Can you work these out from the model? Positions are in its coordinate system, mm. Round coordinates to 2 decimals unless told otherwise and drop trailing zeros. Write each loop counter-clockwise with the first axis right and the second up, starting at its lowest first coordinate (ties: lowest second). Pieces come first, ordered by that corner, then holes. Notation, with made-up numbers: (-23.5, -39.5) -> (4.5, -39.5) arc R22 ccw to (4.5, -31.5) -> close; hole circle Ø7 at (2, 13). An arc over 180 degrees is marked (long way). Write item = value, one per line. Start each with the question number.
1) Imagine slicing it at A-A, the plane y = -115.57. Please give me the cut outline in (x, z) (3 decimals).
2) Imagine slicing it at C-C, the plane z = 0.25. State how many separate pieces and enclosed holes the cut face has, then the cut area to 3 significant figures.
3) Thinking about a two-plate mould opening in X: for faces 1 (the face through (109.159, -124.952, 0.789)), 2 (the face through (125, -113, 0)), 3 (the face through (141.82, -104.477, 0.789)), which applies, +X half, -X half, draft (parallel to the pull), parting line (faces both ways), or undercut?
4) Imagine slicing it at B-B, the plane x = 111.76. Please give me the cut outline in (y, z).
5) If I drill on line 1 (X direction, y = -115.57, z = 1.35) (3 decimals); line 2 (X direction, y = -121.5, z = 0.6); line 3 (Y direction, x = 131, z = 0.4), over which ranges is the centre line in solid material (lowest first)?
Autodesk Inventor part; units mm, degrees
ref_plane "Plan YZ" through (0, 0, 0) normal (1, 0, 0) x (0, 1, 0)
ref_plane "Plan XZ" through (0, 0, 0) normal (0, 1, 0) x (-1, 0, 0)
ref_plane "Plan XY" through (0, 0, 0) normal (0, 0, 1) x (1, 0, 0)
sketch "Esquisse1" plane through (0, 0, 0) normal (0, 0, 1) x (1, 0, 0)
  point P0 (0, 0)
sketch "Esquisse6" plane through (0, 0, 0) normal (0, 0, 1) x (1, 0, 0)
  arc A0 (111.379, -99.822) -> (108.204, -102.997) centre (111.379, -102.997) ccw
  line L0 (108.204, -102.997) -> (108.204, -122.682)
  arc A1 (108.204, -122.682) -> (111.379, -125.857) centre (111.379, -122.682) ccw
  line L1 (111.379, -125.857) -> (139.954, -125.857)
  arc A2 (139.954, -125.857) -> (143.129, -122.682) centre (139.954, -122.682) ccw
  line L2 (143.129, -122.682) -> (143.129, -102.997)
  arc A3 (143.129, -102.997) -> (139.954, -99.822) centre (139.954, -102.997) ccw
  line L3 (139.954, -99.822) -> (111.379, -99.822)
  circle A4 centre (120.269, -122.428) radius 0.4
  circle A5 centre (121.539, -119.888) radius 0.4
  circle A6 centre (122.809, -122.428) radius 0.4
  circle A7 centre (124.079, -119.888) radius 0.4
  circle A8 centre (125.349, -122.428) radius 0.4
  circle A9 centre (126.619, -119.888) radius 0.4
  circle A10 centre (127.889, -122.428) radius 0.4
  circle A11 centre (129.159, -119.888) radius 0.4
  circle A12 centre (137.795, -115.57) radius 0.4
  circle A13 centre (127.635, -115.57) radius 0.4
  circle A14 centre (123.825, -115.57) radius 0.4
  circle A15 centre (113.665, -115.57) radius 0.4
  circle A16 centre (131.445, -111.76) radius 0.4
  circle A17 centre (141.605, -111.76) radius 0.4
  circle A18 centre (131.445, -104.14) radius 0.4
  circle A19 centre (141.605, -104.14) radius 0.4
  circle A20 centre (111.76, -111.76) radius 0.4
  circle A21 centre (121.92, -111.76) radius 0.4
  circle A22 centre (111.76, -104.14) radius 0.4
  circle A23 centre (121.92, -104.14) radius 0.4
  circle A24 centre (130.559, -121.688) radius 0.75
  circle A25 centre (139.7, -118.745) radius 1.6
  circle A26 centre (125.476, -102.616) radius 1.6
  circle A27 centre (111.633, -122.174) radius 1.6
extrude "Manette_2019_PCB_Central.kicad_pcb_Contour" add sketch "Esquisse6" along normal blind 1.6
properties part number "Manette_2019_PCB_Central.kicad_pcb_Contour" material "."
Reported:
q1.outline = (108.204, 0) -> (113.265, 0) -> (113.265, 1.6) -> (108.204, 1.6) -> close; (114.065, 0) -> (123.425, 0) -> (123.425, 1.6) -> (114.065, 1.6) -> close; (124.225, 0) -> (127.235, 0) -> (127.235, 1.6) -> (124.225, 1.6) -> close; (128.035, 0) -> (137.395, 0) -> (137.395, 1.6) -> (128.035, 1.6) -> close; (138.195, 0) -> (143.129, 0) -> (143.129, 1.6) -> (138.195, 1.6) -> close
q2.separate_pieces = 1
q2.enclosed_holes = 24
q2.area = 865 mm²
q3.face_1 = -X half
q3.face_2 = draft
q3.face_3 = undercut
q4.outline = (-125.86, 0) -> (-123.77, 0) -> (-123.77, 1.6) -> (-125.86, 1.6) -> close; (-120.58, 0) -> (-112.16, 0) -> (-112.16, 1.6) -> (-120.58, 1.6) -> close; (-111.36, 0) -> (-104.54, 0) -> (-104.54, 1.6) -> (-111.36, 1.6) -> close; (-103.74, 0) -> (-99.82, 0) -> (-99.82, 1.6) -> (-103.74, 1.6) -> close
q5.line_1 = 108.204 to 113.265, 114.065 to 123.425, 124.225 to 127.235, 128.035 to 137.395, 138.195 to 143.129
q5.line_2 = 108.2 to 110.18, 113.08 to 129.83, 131.29 to 143.13
q5.line_3 = -125.86 to -122.29, -121.08 to -99.82
